Read the model definition and answer for the solid it produces. Units are mm, in the model's axes. Coordinates: 2 decimals unless noted, no trailing zeros. Write each loop counter-clockwise with the first axis right and the second up, starting at its lowest first coordinate (ties: lowest second). Pieces come first, ordered by that corner, then holes.
(1) Find the intervals of material crossed by probe 1 along X at (y, z) = (37, 0.7); probe 2 along Y at (x, z) = (-5.2, 2.3); probe 3 along Y at (x, z) = (-11.5, 1.1), in increasing order.
(2) Section C-C on x = 5.2 is taken. Write down the section's boundary in (y, z).
(3) Section B-B on y = -6 is taken. Write down the section's boundary in (x, z), then the cut area to 3 significant figures.
(4) Given pin 1 (1 mm diameter, centred on y = 22, z = 1, fed in from +X); pin 2 (9.5 mm diameter, centred on x = 0, y = 0, fed in from +Z), each flat-ended and moving along its own axis, determine where each tip first touches the part or whether it passes through.
(5) Section D-D on z = 2 is taken. State how many separate pieces and enclosed holes the cut face has, then the cut area to 3 significant figures.
(6) Section A-A on x = 14.5 is taken. Write down the section's boundary in (y, z), then the cut area to 3 significant figures.
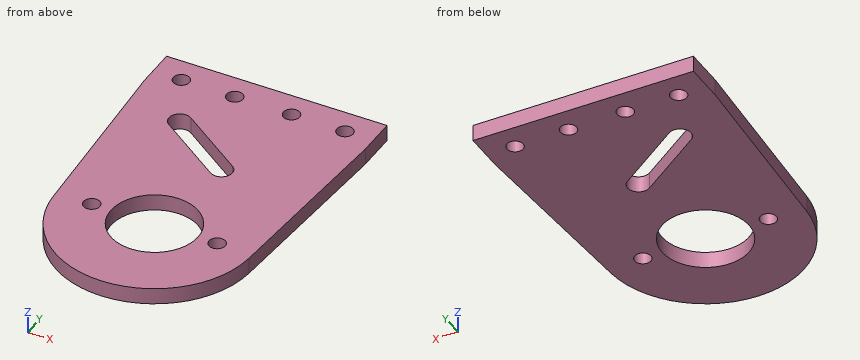
from build123d import *

# Parameters (mm, degrees)
SKETCH1_R               = 7.95
SKETCH1_R_2             = 1.5
MAIN_BODY_LINK_B2_DEPTH = 3
CUT_EXTRUDE1_REACH      = 48.409
SKETCH2_R               = 1.5
CUT_EXTRUDE2_DEPTH      = 47.408691448


with BuildPart() as part:
    # Sketch1 → Main Body Link B2 (new body)
    with BuildSketch(Plane.XY):
        with BuildLine():
            Line((0, 41.674052381), (20.2, 41.674052381))
            Line((20.2, 41.674052381), (20.2, 34.274052381))
            Line((20.2, 34.274052381), (17.964224051, -1.134307826))
            ThreePointArc((17.964224051, -1.134307826), (0, -18), (-17.964224051, -1.134307826))
            Line((-17.964224051, -1.134307826), (-20.2, 34.274052381))
            Line((-20.2, 34.274052381), (-20.2, 41.674052381))
            Line((-20.2, 41.674052381), (0, 41.674052381))
        make_face()
        Circle(SKETCH1_R, mode=Mode.SUBTRACT)
        with Locations((-15, 37.024052381)):
            Circle(SKETCH1_R_2, mode=Mode.SUBTRACT)
        with Locations((-5.2, 37.024052381)):
            Circle(SKETCH1_R_2, mode=Mode.SUBTRACT)
        with Locations((5.2, 37.024052381)):
            Circle(SKETCH1_R_2, mode=Mode.SUBTRACT)
        with Locations((15, 37.024052381)):
            Circle(SKETCH1_R_2, mode=Mode.SUBTRACT)
    extrude(amount=MAIN_BODY_LINK_B2_DEPTH)

    # Sketch2 → Cut-Extrude1 (cut, up to next)
    with BuildSketch(Plane.XY.offset(3), mode=Mode.PRIVATE) as cut_extrude1_sk1:
        with Locations((-11.5, 0)):
            Circle(SKETCH2_R)
    cut_extrude1_tool1 = extrude(cut_extrude1_sk1.sketch, amount=-CUT_EXTRUDE1_REACH, mode=Mode.PRIVATE) & part.part
    # Sketch2 → Cut-Extrude1 (cut, up to next)
    with BuildSketch(Plane.XY.offset(3), mode=Mode.PRIVATE) as cut_extrude1_sk2:
        with Locations((11.5, 0)):
            Circle(SKETCH2_R)
    cut_extrude1_tool2 = extrude(cut_extrude1_sk2.sketch, amount=-CUT_EXTRUDE1_REACH, mode=Mode.PRIVATE) & part.part
    add(cut_extrude1_tool1.solids().sort_by_distance((-11.5, 0, 3))[0], mode=Mode.SUBTRACT)
    add(cut_extrude1_tool2.solids().sort_by_distance((11.5, 0, 3))[0], mode=Mode.SUBTRACT)

    # Sketch3 → Cut-Extrude2 (cut, through all)
    with BuildSketch(Plane.XY.offset(3)):
        with BuildLine():
            Line((-8.682671659, 28.521221325), (3.604609006, 19.91757478))
            ThreePointArc((3.604609006, 19.91757478), (4.095760221, 17.132117818), (1.31030326, 16.640966602))
            Line((1.31030326, 16.640966602), (-10.976977404, 25.244613148))
            ThreePointArc((-10.976977404, 25.244613148), (-11.46812862, 28.030070109), (-8.682671659, 28.521221325))
        make_face()
    extrude(amount=-CUT_EXTRUDE2_DEPTH, mode=Mode.SUBTRACT)


solid = part.part
Response:
1. probe 1: x = -20.2 to -16.5, -13.5 to -6.7, -3.7 to 3.7, 6.7 to 13.5, 16.5 to 20.2
1. probe 2: y = -17.23 to -6.01, 6.01 to 21.2, 26.08 to 35.52, 38.52 to 41.67
1. probe 3: y = -13.85 to -1.5, 1.5 to 25.78, 27.98 to 41.67
2. outline: (-17.23, 0) - (-6.01, 0) - (-6.01, 3) - (-17.23, 3) - close; (6.01, 0) - (35.52, 0) - (35.52, 3) - (6.01, 3) - close; (38.52, 0) - (41.67, 0) - (41.67, 3) - (38.52, 3) - close
3. outline: (-16.97, 0) - (-5.22, 0) - (-5.22, 3) - (-16.97, 3) - close; (5.22, 0) - (16.97, 0) - (16.97, 3) - (5.22, 3) - close
3. area: 70.5 mm2
4. pin 1: stops at x = 19.46
4. pin 2: passes through
5. separate pieces: 1
5. enclosed holes: 8
5. area: 1,800 mm2
6. outline: (-10.67, 0) - (35.61, 0) - (35.61, 3) - (-10.67, 3) - close; (38.44, 0) - (41.67, 0) - (41.67, 3) - (38.44, 3) - close
6. area: 149 mm2
